```python
from build123d import *

# Parameters (mm, degrees)
BOSS_EXTRUDE1_DEPTH      = 32
BOSS_EXTRUDE1_DEPTH_BACK = 29
SKETCH1_R                = 10
CUT_EXTRUDE1_START       = -32
CUT_EXTRUDE1_DEPTH       = 32
SKETCH3_R                = 5
BOSS_EXTRUDE2_DEPTH      = 2
SKETCH4_R                = 2
BOSS_EXTRUDE3_DEPTH      = 13
CUT_EXTRUDE2_START       = -8
CUT_EXTRUDE2_DEPTH       = 8


with BuildPart() as part:
    # Sketch1 → Boss-Extrude1 (new, two sides: drawn at the far end of the back side and taken through both)
    with BuildSketch(Plane.XY.offset(-BOSS_EXTRUDE1_DEPTH_BACK)):
        Circle(SKETCH1_R)
    extrude(amount=BOSS_EXTRUDE1_DEPTH + BOSS_EXTRUDE1_DEPTH_BACK)

    # Sketch2 → Cut-Extrude1 (cut)
    with BuildSketch(Plane.XY.offset(32).offset(CUT_EXTRUDE1_START)):
        with BuildLine():
            Line((6.31961233, -7.75), (-6.31961233, -7.75))
            ThreePointArc((-6.31961233, -7.75), (0, -10), (6.31961233, -7.75))
        make_face()
        with BuildLine():
            ThreePointArc((6.31961233, 7.75), (0, 10), (-6.31961233, 7.75))
            Line((-6.31961233, 7.75), (6.31961233, 7.75))
        make_face()
    extrude(amount=CUT_EXTRUDE1_DEPTH, mode=Mode.SUBTRACT)

    # Sketch3 → Boss-Extrude2 (add)
    with BuildSketch(Plane(origin=(0, 0, -29), x_dir=(-1, 0, 0), z_dir=(0, 0, -1))):
        Circle(SKETCH3_R)
    extrude(amount=BOSS_EXTRUDE2_DEPTH)

    # Sketch4 → Boss-Extrude3 (add)
    with BuildSketch(Plane(origin=(0, 0, -31), x_dir=(-1, 0, 0), z_dir=(0, 0, -1))):
        with Locations(Location((0, 0, 0), (0, 0, 180))):
            Circle(SKETCH4_R)
    extrude(amount=BOSS_EXTRUDE3_DEPTH)

    # Sketch5 → Cut-Extrude2 (cut)
    with BuildSketch(Plane(origin=(0, 0, -44), x_dir=(-1, 0, 0), z_dir=(0, 0, -1)).offset(CUT_EXTRUDE2_START)):
        with BuildLine():
            Line((-1.322875656, 1.5), (1.322875656, 1.5))
            ThreePointArc((1.322875656, 1.5), (0, 2), (-1.322875656, 1.5))
        make_face()
    extrude(amount=CUT_EXTRUDE2_DEPTH, mode=Mode.SUBTRACT)


solid = part.part
```
Work out the finished part from the listing and answer in its coordinate system (mm). A direction names the side the tool comes from. Give positions to 0.01 mm unless a question says otherwise; leave off trailing zeros. Write each loop counter-clockwise with the first axis right and the second up, starting at its lowest first coordinate (ties: lowest second). Pieces come first, ordered by that corner, then holes.
(1) The part is cut by section C-C on z = 27.5. Write down the section's boundary in (x, y), plus the area to 3 significant figures.
Final values:
outline: (-6.32, -7.75) - (6.32, -7.75) arc R10 ccw to (6.32, 7.75) - (-6.32, 7.75) arc R10 ccw to start
area: 275 mm2
(2) The part is cut by section A-A on x = 0. Write down the section's boundary in (y, z), plus the area to 3 significant figures.
Final values:
outline: (-10, -29) - (-5, -29) - (-5, -31) - (-2, -31) - (-2, -44) - (1.5, -44) - (1.5, -36) - (2, -36) - (2, -31) - (5, -31) - (5, -29) - (10, -29) - (10, 0) - (7.75, 0) - (7.75, 32) - (-7.75, 32) - (-7.75, 0) - (-10, 0) - close
area: 1,140 mm2
(3) Flat-ended cylindrical pins translate along their axes: pin 1 Ø1 at (x, y) = (4, 7.5) entering from -Z; pin 2 Ø8 at (x, z) = (6.5, 11) entering from -Y; pin 3 Ø0.7 at (x, y) = (2.5, 9) entering from +Z. Find the tip coordinate at first contact, or state that the pin passes through.
Final values:
pin 1: stops at z = -29
pin 2: stops at y = -7.75
pin 3: stops at z = 0
(4) The part is cut by section B-B on y = 0. Write down the section's boundary in (x, z), plus the area to 3 significant figures.
Final values:
outline: (-10, -29) - (-5, -29) - (-5, -31) - (-2, -31) - (-2, -44) - (2, -44) - (2, -31) - (5, -31) - (5, -29) - (10, -29) - (10, 32) - (-10, 32) - close
area: 1,290 mm2
(5) Which of the six approach directions +Z, -Z, +X, -X, +Y, -Y give full straight-line access (tool end or side, diameter ignored) to faces 1 (the cylindrical face through (0, -2, -37)), 2 (the flat face through (0, 9, 0)), 3 (the flat face through (0, 1.5, -40)), 4 (the flat face through (0, -7.75, 16))?
Final values:
face 1: -Z
face 2: +Z, +X, -X, +Y
face 3: -Z, +X, -X, +Y
face 4: +Z, +X, -X, -Y
(6) Straight lines are drawn through the part: line 1 (Y direction, x = 5.25, z = 3.5); line 2 (Z direction, x = 6, y = 5.5); line 3 (Y direction, x = -0.5, z = -15.5). For each, find the intervals that lie inside material, in ascending order.
Final values:
line 1: y = -7.75 to 7.75
line 2: z = -29 to 32
line 3: y = -9.99 to 9.99
(7) The part is cut by section D-D on x = -8. Write down the section's boundary in (y, z), plus the area to 3 significant figures.
Final values:
outline: (-6, -29) - (6, -29) - (6, 32) - (-6, 32) - close
area: 732 mm2
